Job drawing, mm, ordinate dimensions from the low corner. One solid piece. Round coordinates to 2 decimals unless told otherwise and drop trailing zeros. Loops run counter-clockwise (first coordinate to the right, second up) from the corner with the lowest first, then second, coordinate; pieces in that order, holes last. Notation, with made-up numbers: M -7.5,27 L 49.5,27 A23 ccw 49.5,40 Z; hole C 72.25,65.25 d11. An arc over 180 degrees is marked long. Put each result on its own line as item: value. Start each with the question number.
1) Slice it at C-C on z = 15.75. Give the cut face in (x, y).
2) Slice it at B-B on x = 4. Give the cut face in (y, z).
3) Slice it at A-A on y = 4.75. Give the cut face in (x, z).
4) Drop flat-ended pins along their axis: pin 1 Ø5.5 at (x, z) = (13.5, 17.5) entering from +Y; pin 2 Ø1.2 at (x, y) = (29, 1) entering from +Z; pin 3 Ø2 at (y, z) = (0.5, 3) entering from -X; pin 4 Ø1.5 at (x, y) = (7.5, 1.5) entering from +Z. Give the stop position or say it passes through.
5) Pull direction X, two halves, no side cores. Call the marked faces 1, 2 and 3: +X half, -X half, draft (parallel to the pull), parting line (faces both ways), or undercut.
6) Probe line 1 along X through (y, z) = (5.25, 11.5); line 2 along Z through (x, y) = (20.5, 4.25); line 3 along Z through (x, y) = (25.5, 2.25). List the from-to ranges inside material, lowest first.
7) Slice it at D-D on x = 31.5. Give the cut face in (y, z).
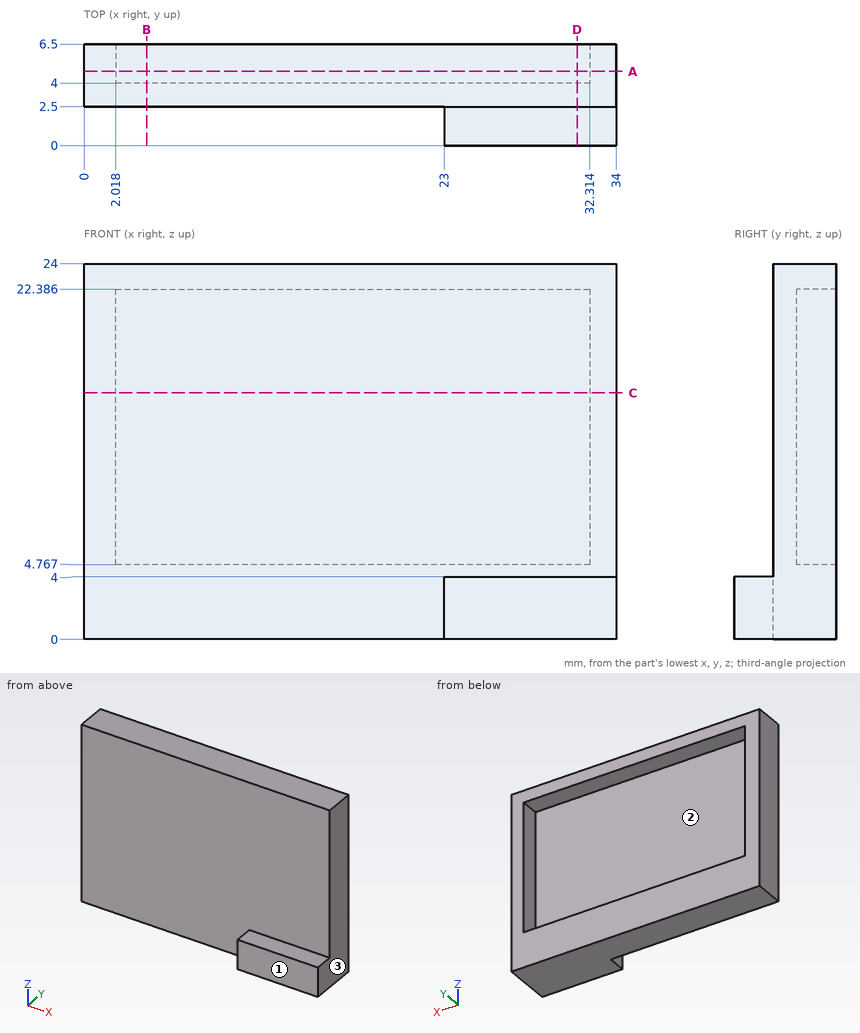
Recorded:
1. outline: M 0,2.5 L 34,2.5 L 34,6.5 L 32.31,6.5 L 32.31,4 L 2.02,4 L 2.02,6.5 L 0,6.5 Z
2. outline: M 2.5,0 L 6.5,0 L 6.5,4.77 L 4,4.77 L 4,22.39 L 6.5,22.39 L 6.5,24 L 2.5,24 Z
3. outline: M 0,0 L 34,0 L 34,24 L 0,24 Z; hole M 2.02,4.77 L 32.31,4.77 L 32.31,22.39 L 2.02,22.39 Z
4. pin 1: stops at y = 4
4. pin 2: stops at z = 4
4. pin 3: stops at x = 23
4. pin 4: passes through
5. face 1: draft
5. face 2: undercut
5. face 3: +X half
6. line 1: x = 0 to 2.02, 32.31 to 34
6. line 2: z = 0 to 4.77, 22.39 to 24
6. line 3: z = 0 to 4
7. outline: M 0,0 L 6.5,0 L 6.5,4.77 L 4,4.77 L 4,22.39 L 6.5,22.39 L 6.5,24 L 2.5,24 L 2.5,4 L 0,4 Z
